Read the model definition and answer for the solid it produces. Units are mm, in the model's axes. A direction names the side the tool comes from. Coordinates: 2 decimals unless noted, no trailing zeros. Loops run counter-clockwise (first coordinate to the right, second up) from the corner with the lowest first, then second, coordinate; pieces in that order, holes last. Notation, with made-up numbers: (-2.75, 30.5) -> (10.25, 30.5) arc R19 ccw to (10.25, 62.5) -> close; hole circle Ø3 at (27.5, 71.5). An arc over 180 degrees is marked (long way). Answer in a Markdown table with one row per item.
```python
from build123d import *

# Parameters (mm, degrees)
F0_W     = 76.2
F0_H     = 57.15
F1_DEPTH = 6.35
F2_R     = 22.225
F3_DEPTH = 6.35
F5_D     = 6.7564
F7_D     = 1.5875
F7_DEPTH = 6.35
F7_TIP   = 0.4769331164


with BuildPart() as f1:
    # F0 (on Top) → F1 (new body)
    with BuildSketch(Plane.XY):
        with Locations((38.1, 28.575)):
            Rectangle(F0_W, F0_H)
    extrude(amount=F1_DEPTH)

    # F2 (on face) → F3 (join)
    with BuildSketch(Plane.XY.offset(6.35)):
        with Locations((38.1, 28.575)):
            Circle(F2_R)
    extrude(amount=F3_DEPTH)

    # F5 (through all)
    with Locations(Plane.XY.offset(6.35)):
        with Locations((5.08, 5.08), (5.08, 52.07), (71.12, 52.07), (71.12, 5.08)):
            Hole(F5_D / 2)

    # F7
    with Locations(Plane.XY.offset(12.7)):
        with Locations((38.1, 45.72), (25.9766542366, 40.6983457634), (20.955, 28.575), (25.9766542366, 16.4516542366), (38.1, 11.43), (50.2233457634, 16.4516542366), (55.245, 28.575), (50.2233457634, 40.6983457634), (42.960079591, 40.3082700629), (33.239920409, 40.3082700629), (26.3667299371, 33.435079591), (26.3667299371, 23.714920409), (33.239920409, 16.8417299371), (42.960079591, 16.8417299371), (49.8332700629, 23.714920409), (49.8332700629, 33.435079591), (38.1, 34.925), (31.75, 28.575), (38.1, 22.225), (44.45, 28.575), (38.1, 28.575)):
            Hole(F7_D / 2, depth=F7_DEPTH)
            with Locations((0, 0, -(F7_DEPTH + F7_TIP / 2))):  # 118° drill point
                Cone(0, F7_D / 2, F7_TIP, mode=Mode.SUBTRACT)


solid = f1.part
```
1. A cutting plane is placed at B-B on y = 5.08. Give the vertices of the cut face in (x, z).
A:
| item | result |
|---|---|
| outline | (0, 0) -> (1.7, 0) -> (1.7, 6.35) -> (0, 6.35) -> close; (8.46, 0) -> (67.74, 0) -> (67.74, 6.35) -> (8.46, 6.35) -> close; (74.5, 0) -> (76.2, 0) -> (76.2, 6.35) -> (74.5, 6.35) -> close |
2. Given pin 1 Ø1.4 at (x, y) = (49.83, 23.71) entering from +Z; pin 2 Ø1.5 at (y, z) = (23, 11.5) entering from -X; pin 3 Ø4 at (y, z) = (23.5, 8.5) entering from -X, each flat-ended and moving along its own axis, determine where each tip first touches the part or whether it passes through.
A:
| item | result |
|---|---|
| pin 1 | stops at z = 6.3 |
| pin 2 | stops at x = 16.41 |
| pin 3 | stops at x = 16.09 |
3. The mould has two halves that part along Y. Classify faces 1 (the conical face through (37.991, 11.346, 5.956)), 2 (the flat face through (76.2, 28, 3)), 3 (the cylindrical face through (50.048, 47.315, 9.481)): pulls with the +Y half, pulls with the -Y half, needs draft (parallel to the pull), parting line crosses it, or undercut.
A:
| item | result |
|---|---|
| face 1 | undercut |
| face 2 | needs draft |
| face 3 | parting line crosses it |
4. A cutting plane is placed at C-C on z = 5. Give the vertices of the cut face in (x, y).
A:
| item | result |
|---|---|
| outline | (0, 0) -> (76.2, 0) -> (76.2, 57.15) -> (0, 57.15) -> close; hole circle Ø6.76 at (5.08, 5.08); hole circle Ø6.76 at (5.08, 52.07); hole circle Ø6.76 at (71.12, 5.08); hole circle Ø6.76 at (71.12, 52.07) |
5. A cutting plane is placed at D-D on y = 37. Give the vertices of the cut face in (x, z).
A:
| item | result |
|---|---|
| outline | (0, 0) -> (76.2, 0) -> (76.2, 6.35) -> (58.67, 6.35) -> (58.67, 12.7) -> (17.53, 12.7) -> (17.53, 6.35) -> (0, 6.35) -> close |
6. A cutting plane is placed at A-A on x = 5.08. Give the vertices of the cut face in (y, z).
A:
| item | result |
|---|---|
| outline | (0, 0) -> (1.7, 0) -> (1.7, 6.35) -> (0, 6.35) -> close; (8.46, 0) -> (48.69, 0) -> (48.69, 6.35) -> (8.46, 6.35) -> close; (55.45, 0) -> (57.15, 0) -> (57.15, 6.35) -> (55.45, 6.35) -> close |
7. A tool of negligible diameter and unlimited length cuts with its end or side. For faces 4 (the cylindrical face through (26.149, 39.923, 9.481)), 5 (the cylindrical face through (67.999, 3.786, 3.131)), from which of +Z, -Z, +X, -X, +Y, -Y can it reach the whole face along a straight path? Write none if from no direction.
A:
| item | result |
|---|---|
| face 4 | +Z |
| face 5 | +Z, -Z |
8. Find the intervals of material crossed by probe 1 along Y at (x, z) = (71.12, 3.25); probe 2 along Y at (x, z) = (69, 5.5); probe 3 along Z at (x, y) = (8, 9), in increasing order.
A:
| item | result |
|---|---|
| probe 1 | y = 0 to 1.7, 8.46 to 48.69, 55.45 to 57.15 |
| probe 2 | y = 0 to 2.45, 7.71 to 49.44, 54.7 to 57.15 |
| probe 3 | z = 0 to 6.35 |
